```python
from build123d import *

# Parameters (mm, degrees)
SKETCH1_R           = 23.5
BOSS_EXTRUDE1_DEPTH = 32.8
SKETCH5_W           = 18.1
SKETCH5_H           = 47
CUT_EXTRUDE1_DEPTH  = 13.8
SKETCH6_R           = 23.5
BOSS_EXTRUDE2_DEPTH = 1.5
CUT_EXTRUDE5_DEPTH  = 1.5


with BuildPart() as part:
    # Sketch1 → Boss-Extrude1 (new body)
    with BuildSketch(Plane.XY):
        Circle(SKETCH1_R)
    extrude(amount=BOSS_EXTRUDE1_DEPTH)

    # Sketch5 → Cut-Extrude1 (cut)
    with BuildSketch(Plane(origin=(0, 0, 0), x_dir=(-1, 0, 0), z_dir=(0, 0, -1))):
        Rectangle(SKETCH5_W, SKETCH5_H)
    extrude(amount=-CUT_EXTRUDE1_DEPTH, mode=Mode.SUBTRACT)

    # Sketch6 → Boss-Extrude2 (add)
    with BuildSketch(Plane.XY):
        Circle(SKETCH6_R)
    extrude(amount=-BOSS_EXTRUDE2_DEPTH)

    # Sketch8 → Cut-Extrude5 (cut)
    with BuildSketch(Plane(origin=(0, 0, -1.5), x_dir=(-1, 0, 0), z_dir=(0, 0, -1))):
        with BuildLine():
            Line((-9.05, 8.2), (9.05, 8.2))
            Line((9.05, 8.2), (9.05, -21.687496398))
            ThreePointArc((9.05, -21.687496398), (0, -23.5), (-9.05, -21.687496398))
            Line((-9.05, -21.687496398), (-9.05, 8.2))
        make_face()
    extrude(amount=-CUT_EXTRUDE5_DEPTH, mode=Mode.SUBTRACT)


solid = part.part
```
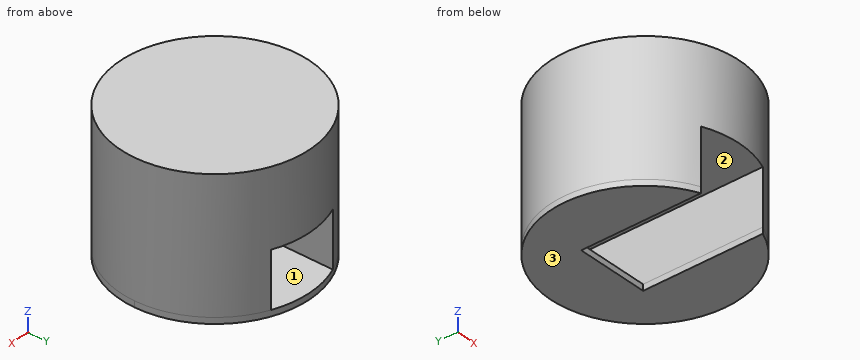
Design review of the part built by this model. Coordinates are the model's own, in mm. Face numbers are marked on the shaded views. Coordinates: 2 decimals unless noted, no trailing zeros. Order: outer loops, then holes, each group sorted by start corner. A loop starts at its lowest first (then second) coordinate and runs counter-clockwise, first axis right, second up.
1) Wall thickness on line 1 along X through (y, z) = (0, 13); line 2 along Z through (x, y) = (-1, 19.5); line 3 along X through (y, z) = (-18.5, 2.5): over which ranges is each line inside the solid? List them lowest first.
2) Take a section at A-A, the plane x = 0. Give the boundary of the cut face in (y, z).
3) Take a section at C-C, the plane y = -13.5. Give the boundary of the cut face in (x, z).
4) Clearance check with flat-ended pins moving along their axes: pin 1 (0.8 mm diameter, centred on x = -4, z = -1, fed in from -Y); pin 2 (8 mm diameter, centred on x = 16.5, z = 13, fed in from -Y); pin 3 (11 mm diameter, centred on y = -0.5, z = 5.5, fed in from +X); pin 4 (6 mm diameter, centred on y = 4, z = 25.5, fed in from -X). State where each tip first meets the part, or that it passes through.
5) Take a section at B-B, the plane y = 13. Give the boundary of the cut face in (x, z).
6) Mouldability with a two-part tool opening along X and no side actions: class the marked faces 1, 2 and 3 as +X half, -X half, draft (parallel to the pull), parting line (faces both ways), or undercut.
7) Take a section at D-D, the plane z = 20. Give the boundary of the cut face in (x, y).
Returned:
1. line 1: x = -23.5 to -9.05, 9.05 to 23.5
1. line 2: z = -1.5 to 0, 13.8 to 32.8
1. line 3: x = -14.49 to -9.05, 9.05 to 14.49
2. outline: (-23.5, 13.8) - (23.5, 13.8) - (23.5, 32.8) - (-23.5, 32.8) - close; (8.2, -1.5) - (23.5, -1.5) - (23.5, 0) - (8.2, 0) - close
3. outline: (-19.24, -1.5) - (-9.05, -1.5) - (-9.05, 13.8) - (9.05, 13.8) - (9.05, -1.5) - (19.24, -1.5) - (19.24, 32.8) - (-19.24, 32.8) - close
4. pin 1: stops at y = 8.2
4. pin 2: stops at y = -19.9
4. pin 3: stops at x = 23.5
4. pin 4: stops at x = -23.48
5. outline: (-19.58, -1.5) - (19.58, -1.5) - (19.58, 32.8) - (-19.58, 32.8) - close; hole (-9.05, 0) - (9.05, 0) - (9.05, 13.8) - (-9.05, 13.8) - close
6. face 1: undercut
6. face 2: undercut
6. face 3: draft
7. outline: circle Ø47 at (0, 0)
